```python
from build123d import *

# Parameters (mm, degrees)
F0_R     = 12.5
F1_DEPTH = 0.1016


with BuildPart() as f1:
    # F0 (on Top) → F1 (new body)
    with BuildSketch(Plane.XY):
        Circle(F0_R)
        with BuildLine():
            Line((2.648541, 9.655839), (0.856066, 1.554615))
            Line((0.856066, 1.554615), (6.743845, 7.400713))
            ThreePointArc((6.743845, 7.400713), (7.450947, 7.398201), (7.448436, 6.691099))
            Line((7.448436, 6.691099), (1.560657, 0.845001))
            Line((1.560657, 0.845001), (9.674411, 2.579878))
            ThreePointArc((9.674411, 2.579878), (10.267905, 2.195477), (9.883504, 1.601982))
            Line((9.883504, 1.601982), (1.76975, -0.132895))
            Line((1.76975, -0.132895), (9.53342, -3.06005))
            ThreePointArc((9.53342, -3.06005), (9.824876, -3.704296), (9.18063, -3.995752))
            Line((9.18063, -3.995752), (1.41696, -1.068598))
            Line((1.41696, -1.068598), (6.365635, -7.728434))
            ThreePointArc((6.365635, -7.728434), (6.262518, -8.427981), (5.56297, -8.324864))
            Line((5.56297, -8.324864), (0.614295, -1.665028))
            Line((0.614295, -1.665028), (1.176807, -9.943094))
            ThreePointArc((1.176807, -9.943094), (0.711855, -10.475842), (0.179107, -10.01089))
            Line((0.179107, -10.01089), (-0.383404, -1.732824))
            Line((-0.383404, -1.732824), (-4.38565, -9.000893))
            ThreePointArc((-4.38565, -9.000893), (-5.064817, -9.197697), (-5.261621, -8.518529))
            Line((-5.261621, -8.518529), (-1.259375, -1.25046))
            Line((-1.259375, -1.25046), (-8.555694, -5.200972))
            ThreePointArc((-8.555694, -5.200972), (-9.233446, -4.999348), (-9.031822, -4.321596))
            Line((-9.031822, -4.321596), (-1.735504, -0.371084))
            Line((-1.735504, -0.371084), (-10.009365, 0.250222))
            ThreePointArc((-10.009365, 0.250222), (-10.47052, 0.786259), (-9.934483, 1.247414))
            Line((-9.934483, 1.247414), (-1.660622, 0.626108))
            Line((-1.660622, 0.626108), (-8.285134, 5.621971))
            ThreePointArc((-8.285134, 5.621971), (-8.383279, 6.322234), (-7.683016, 6.420379))
            Line((-7.683016, 6.420379), (-1.058504, 1.424516))
            Line((-1.058504, 1.424516), (-3.930431, 9.208785))
            ThreePointArc((-3.930431, 9.208785), (-3.634405, 9.850944), (-2.992246, 9.554918))
            Line((-2.992246, 9.554918), (-0.120319, 1.77065))
            Line((-0.120319, 1.77065), (1.672156, 9.871874))
            ThreePointArc((1.672156, 9.871874), (2.268366, 10.252049), (2.648541, 9.655839))
        make_face(mode=Mode.SUBTRACT)
    extrude(amount=F1_DEPTH)


solid = f1.part
```
Geometry check sheet. Reference: the model listing, model coordinates, mm. Coordinates: 2 decimals unless noted, no trailing zeros. Write each loop counter-clockwise with the first axis right and the second up, starting at its lowest first coordinate (ties: lowest second). Pieces come first, ordered by that corner, then holes. Notation, with made-up numbers: M -13.75,7 L -5.75,7 A27 ccw -5.75,41 Z; hole C 77.5,85.25 d2. An arc over 180 degrees is marked long. Use one line per item in the form item = value. Start each with the question number.
1) Thickness scan on probe 1 along X at (y, z) = (5.5, 0.05); probe 2 along X at (y, z) = (9.75, 0.05); probe 3 along X at (y, z) = (9, 0.05). Record the ranges inside material, lowest first. Write a range as from..to.
2) Section check D-D on x = 11. Enter the section's corners in (y, z), and give its area (3 significant figures).
3) Section check B-B on y = 8. Enter the section's corners in (x, z).
4) Section check C-C on x = 2.25. Enter the section's corners in (y, z), and give its area (3 significant figures).
Responses:
q1.probe_1 = -11.22..-8.12, -6.46..-2.56, -1.5..0.7, 1.73..4.83, 6.25..11.22
q1.probe_2 = -7.82..-3.8, -3.12..1.65, 2.66..7.82
q1.probe_3 = -8.67..-3.85, -2.79..1.48, 2.5..8.67
q2.outline = M -5.94,0 L 5.94,0 L 5.94,0.1 L -5.94,0.1 Z
q2.area = 1.21 mm2
q3.outline = M -9.6,0 L -3.48,0 L -3.48,0.1 L -9.6,0.1 Z; M -2.42,0 L 1.26,0 L 1.26,0.1 L -2.42,0.1 Z; M 2.28,0 L 9.6,0 L 9.6,0.1 L 2.28,0.1 Z
q4.outline = M -12.3,0 L -3.87,0 L -3.87,0.1 L -12.3,0.1 Z; M -2.19,0 L -1.38,0 L -1.38,0.1 L -2.19,0.1 Z; M -0.31,0 L -0.03,0 L -0.03,0.1 L -0.31,0.1 Z; M 0.99,0 L 1.53,0 L 1.53,0.1 L 0.99,0.1 Z; M 2.94,0 L 7.85,0 L 7.85,0.1 L 2.94,0.1 Z; M 10.26,0 L 12.3,0 L 12.3,0.1 L 10.26,0.1 Z
q4.area = 1.73 mm2
